Check sheet for the drawn part. Datum: minimum x, y, z corner. Units: mm. Give positions to 0.01 mm unless a question says otherwise; leave off trailing zeros. Order: outer loops, then holes, each group sorted by start corner. A loop starts at its lowest first (then second) coordinate and runs counter-clockwise, first axis right, second up.
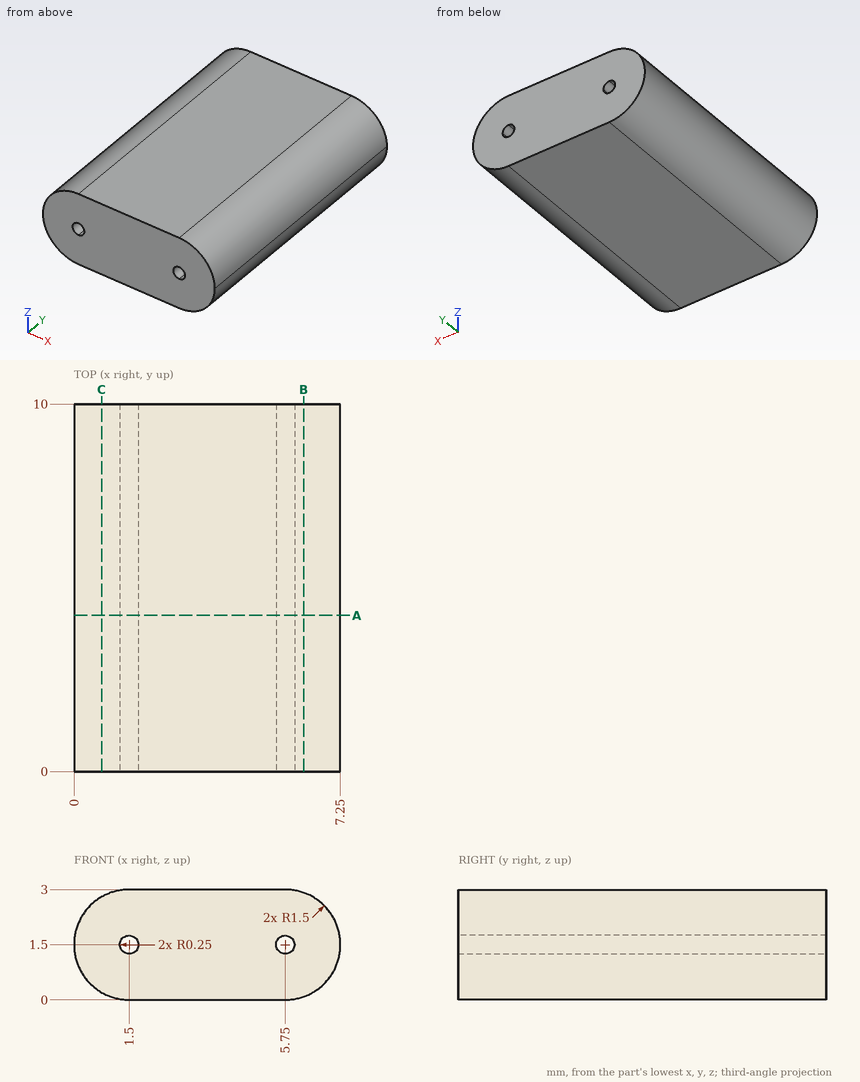
(1) Section check A-A, the plane y = 4.25. Enter the section's corners in (x, z).
Solved:
outline: (1.5, 0) - (5.75, 0) arc R1.5 ccw to (7.25, 1.5) arc R1.5 ccw to (5.75, 3) - (1.5, 3) arc R1.5 ccw to start; hole (1.5, 1.25) arc R0.25 ccw to (1.75, 1.5) arc R0.25 ccw to (1.5, 1.75) arc R0.25 ccw to start; hole (5.75, 1.25) arc R0.25 ccw to (6, 1.5) arc R0.25 ccw to (5.75, 1.75) arc R0.25 ccw to start
(2) Section check C-C, the plane x = 0.75. Enter the section's corners in (y, z).
Solved:
outline: (0, 0.2) - (10, 0.2) - (10, 2.8) - (0, 2.8) - close
(3) Go/stop test with a flat-tipped pin: pin 1 (1.5 mm diameter, centred on y = 3, z = 0.5, fed in from -X). Record where the tip stops, or that it passes through.
Solved:
pin 1: stops at x = 0.02
(4) Scan lines: line 1 (Z direction, x = 6.25, y = 4.75); line 2 (Z direction, x = 7, y = 6); line 3 (X direction, y = 6, z = 0.15). Record each from-to range of solid material in increasing order.
Solved:
line 1: z = 0.09 to 2.91
line 2: z = 0.67 to 2.33
line 3: x = 0.85 to 6.4
(5) Section check B-B, the plane x = 6.25. Enter the section's corners in (y, z), then the cut area to 3 significant figures.
Solved:
outline: (0, 0.09) - (10, 0.09) - (10, 2.91) - (0, 2.91) - close
area: 28.3 mm2
